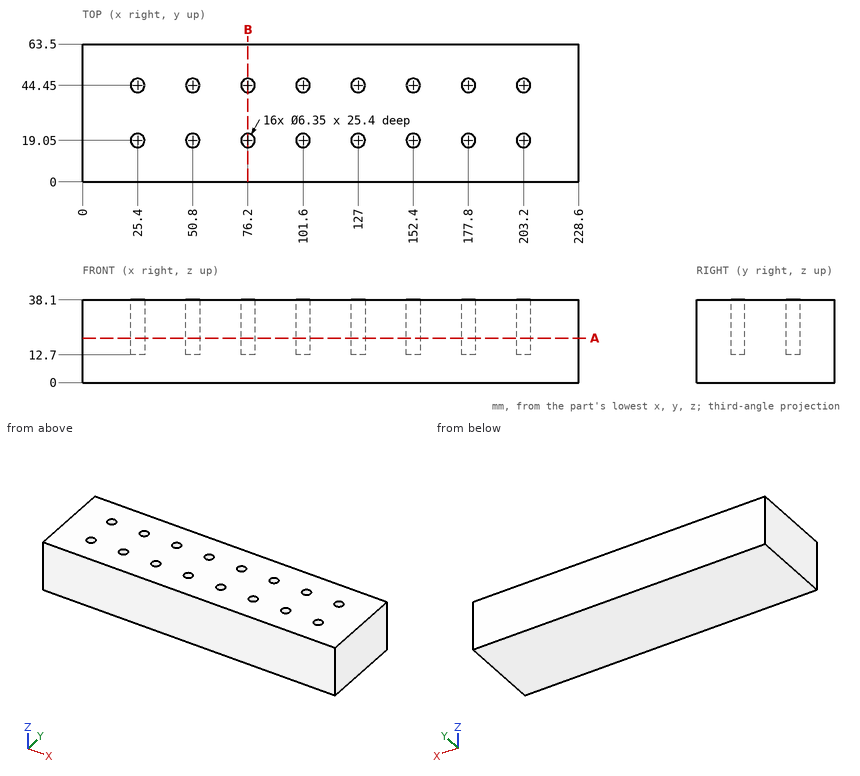
The figure shows three views and two pictorial views of one solid part (mm, origin at its lowest corner). Answer the questions. Give positions to 0.01 mm unless a question says otherwise; leave off trailing zeros. Write each loop counter-clockwise with the first axis right and the second up, starting at its lowest first coordinate (ties: lowest second). Pieces come first, ordered by that corner, then holes. Notation, with made-up numbers: M -12.5,66.5 L 31.5,66.5 A15 ccw 31.5,91.5 Z; hole C 78.5,0.25 d6. An arc over 180 degrees is marked long. One line per item, written item: value. Start each with the question number.
(1) Find section B-B (x = 76.2). Determine the outline of the cut face in (y, z) (3 decimals), plus the area to 3 significant figures.
(2) A flat-ended cylindrical pin translates along its axis: pin 1 Ø4 at (x, y) = (76.2, 19.05) entering from +Z. Find the tip coordinate at first contact, or state that the pin passes through.
(3) Find section A-A (z = 20.5). Give the number of separate pieces and of enclosed holes in the cut face, plus the area to 3 significant figures.
(4) Find the intervals of material crossed by line 1 (Y direction, x = 76.2, z = 29) (3 decimals); line 2 (Y direction, x = 23, z = 33), in increasing order.
Results below:
1. outline: M 0,0 L 63.5,0 L 63.5,38.1 L 47.625,38.1 L 47.625,12.7 L 41.275,12.7 L 41.275,38.1 L 22.225,38.1 L 22.225,12.7 L 15.875,12.7 L 15.875,38.1 L 0,38.1 Z
1. area: 2,100 mm^2
2. pin 1: stops at z = 12.7
3. separate pieces: 1
3. enclosed holes: 16
3. area: 14,000 mm^2
4. line 1: y = 0 to 15.875, 22.225 to 41.275, 47.625 to 63.5
4. line 2: y = 0 to 16.97, 21.13 to 42.37, 46.53 to 63.5
